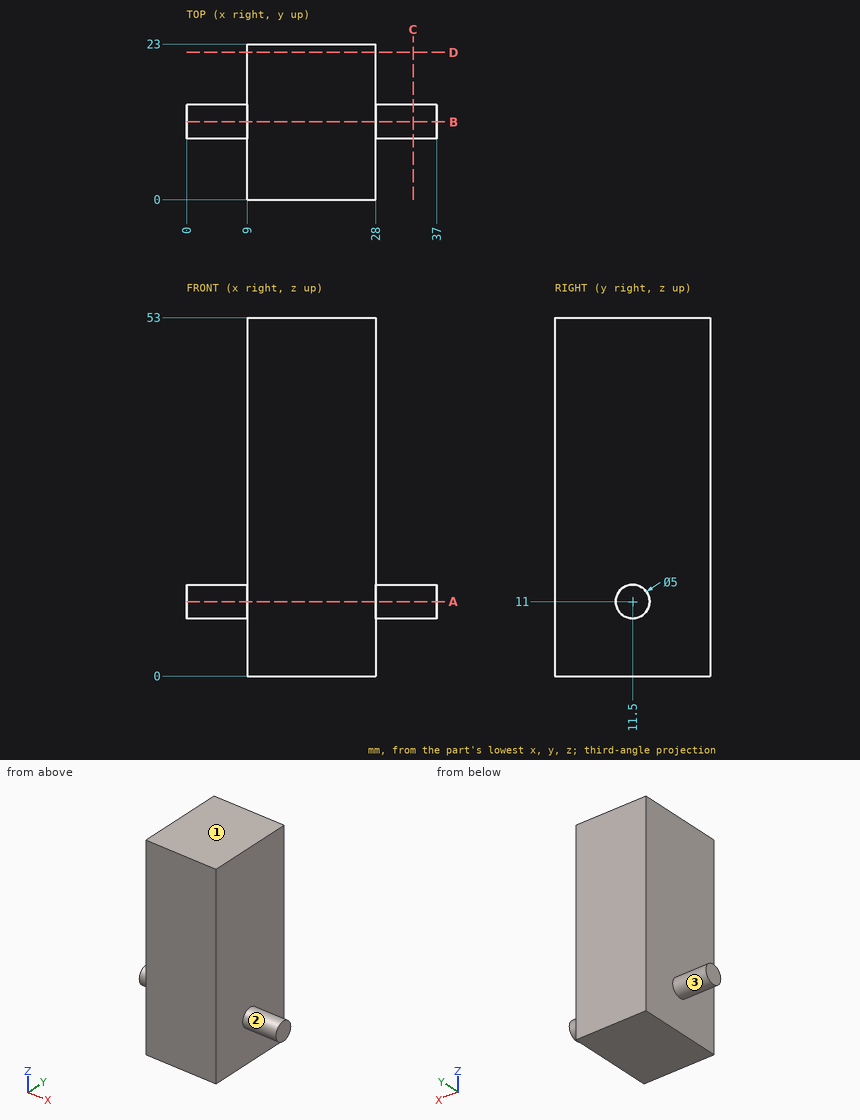
Geometry check sheet. Reference: drawing and pictorial views, mm from the part's lowest x, y, z. A direction names the side the tool comes from. Give positions to 0.01 mm unless a question says otherwise; leave off trailing zeros. Loops run counter-clockwise (first coordinate to the right, second up) from the corner with the lowest first, then second, coordinate; pieces in that order, holes last. Notation, with made-up numbers: M -7,14.25 L 33,14.25 A13 cw 33,37.25 Z; hole C -15,-39.5 d7. An arc over 180 degrees is marked long. Use a Markdown table: item, result. Add a question column.
Q1. Sectioned sample at A-A, the plane z = 11. Record the cut outline in (x, y), then the cut area to 3 significant figures.
Q2. Tool access check on the marked faces 1, 2 and 3. Record the directions out of +Z, -Z, +X, -X, +Y, -Y that give a thin tool (end or side, any length) a straight path to the whole face; none if there is none.
Q3. Sectioned sample at C-C, the plane x = 33.5. Record the cut outline in (y, z).
Q4. Sectioned sample at B-B, the plane y = 11.5. Record the cut outline in (x, z), then the cut area to 3 significant figures.
Q5. Go/stop test with flat-tipped pins: pin 1 (4 mm diameter, centred on x = 18.5, z = 30, fed in from -Y); pin 2 (12 mm diameter, centred on y = 18.5, z = 18, fed in from +X); pin 3 (5 mm diameter, centred on x = 33, y = 15.5, fed in from +Z); pin 4 (6 mm diameter, centred on x = 5.5, y = 3, fed in from +Z). Record where each tip stops, or that it passes through.
Q6. Sectioned sample at D-D, the plane y = 21.75. Record the cut outline in (x, z), then the cut area to 3 significant figures.
Q7. Scan lines: line 1 along X through (y, z) = (5.25, 13); line 2 along Z through (x, y) = (2, 13.5); line 3 along Z through (x, y) = (32, 12.75). Record each from-to range of solid material in increasing order. Write a range as [from, to].
Verdict:
| question | item | result |
|---|---|---|
| 1 | outline | M 0,9 L 9,9 L 9,0 L 28,0 L 28,9 L 37,9 L 37,14 L 28,14 L 28,23 L 9,23 L 9,14 L 0,14 Z |
| 1 | area | 527 mm^2 |
| 2 | face 1 | +Z, +X, -X, +Y, -Y |
| 2 | face 2 | +X |
| 2 | face 3 | -X |
| 3 | outline | C 11.5,11 d5 |
| 4 | outline | M 0,8.5 L 9,8.5 L 9,0 L 28,0 L 28,8.5 L 37,8.5 L 37,13.5 L 28,13.5 L 28,53 L 9,53 L 9,13.5 L 0,13.5 Z |
| 4 | area | 1,100 mm^2 |
| 5 | pin 1 | y = 0 |
| 5 | pin 2 | x = 28 |
| 5 | pin 3 | z = 13 |
| 5 | pin 4 | through |
| 6 | outline | M 9,0 L 28,0 L 28,53 L 9,53 Z |
| 6 | area | 1,010 mm^2 |
| 7 | line 1 | [9, 28] |
| 7 | line 2 | [9.5, 12.5] |
| 7 | line 3 | [8.83, 13.17] |
